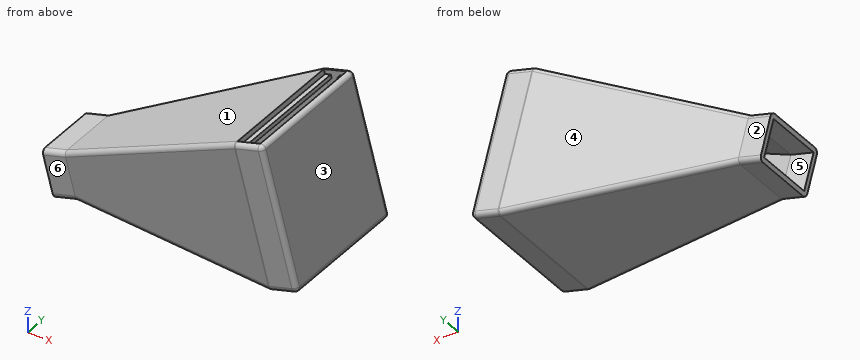
from build123d import *

# Parameters (mm, degrees)
SKETCH037_W             = 110
SKETCH037_H             = 110
PAD002_DEPTH            = 220
POCKET012_DEPTH         = 158
POCKET001_DEPTH         = 158
THICKNESS001_T          = 4
SKETCH014_W             = 110
SKETCH014_H             = 4
POCKET013_DEPTH         = 4
SKETCH016_W             = 3
SKETCH016_H             = 3
PAD022_DEPTH            = 110
SKETCH018_W             = 110
SKETCH018_H             = 16
POCKET014_DEPTH         = 4
SKETCH019_W             = 3
SKETCH019_H             = 5
PAD007_DEPTH            = 110
BODY007_ROLL_ANGLE      = 105
BODY007_PLACEMENT_ANGLE = -90


with BuildPart() as part:
    # Sketch037 → Pad002 (new body)
    with BuildSketch(Plane.XY):
        Rectangle(SKETCH037_W, SKETCH037_H)
    extrude(amount=PAD002_DEPTH)

    # Sketch038 (on Face3 of Pad002) → Pocket012 (cut)
    with BuildSketch(Plane.XZ.offset(55)):
        Polygon((-55, 20), (-25.5, 200), (-25.5, 220), (-55, 220), align=None)
        Polygon((25.5, 220), (55, 220), (55, 20), (25.5, 200), align=None)
    extrude(amount=-POCKET012_DEPTH, mode=Mode.SUBTRACT)

    # Sketch008 (on DatumPlane) → Pocket001 (cut)
    with BuildSketch(Plane.YZ.offset(55)):
        Polygon((-55, 20), (-15.5, 200), (-15.5, 220), (-55, 220), align=None)
        Polygon((15.5, 220), (15.5, 200), (55, 20), (55, 220), align=None)
    extrude(amount=-POCKET001_DEPTH, mode=Mode.SUBTRACT)

    # Thickness001
    thickness001_openings = [part.faces().sort_by_distance(p)[0] for p in [
        (0, 0, 220),
    ]]
    offset(amount=THICKNESS001_T, openings=thickness001_openings)

    # Sketch014 (on Face42 of Thickness001) → Pocket013 (cut)
    with BuildSketch(Plane(origin=(0, 59, 0), x_dir=(-1, 0, 0), z_dir=(0, 1, 0))):
        with Locations((0, 2)):
            Rectangle(SKETCH014_W, SKETCH014_H)
    extrude(amount=-POCKET013_DEPTH, mode=Mode.SUBTRACT)

    # Sketch016 (on Face35 of Pocket013) → Pad022 (join)
    with BuildSketch(Plane(origin=(0, -55, 0), x_dir=(-1, 0, 0), z_dir=(0, 1, 0))):
        with Locations((-53.5, 5.5)):
            Rectangle(SKETCH016_W, SKETCH016_H)
        with Locations((53.5, 5.5)):
            Rectangle(SKETCH016_W, SKETCH016_H)
    extrude(amount=PAD022_DEPTH)

    # Sketch018 (on Face36 of Pad022) → Pocket014 (cut)
    with BuildSketch(Plane(origin=(0, 59, 0), x_dir=(-1, 0, 0), z_dir=(0, 1, 0))):
        with Locations((0, 12)):
            Rectangle(SKETCH018_W, SKETCH018_H)
    extrude(amount=-POCKET014_DEPTH, mode=Mode.SUBTRACT)

    # Sketch019 (on Face49 of Pocket014) → Pad007 (join)
    with BuildSketch(Plane(origin=(55, 0, 0), x_dir=(0, -1, 0), z_dir=(-1, 0, 0))):
        with Locations((-53.5, 17.5)):
            Rectangle(SKETCH019_W, SKETCH019_H)
    extrude(amount=PAD007_DEPTH)


with BuildPart() as part_1:
    # Body007 roll: moved
    add(part.part.rotate(Axis((0, 0, 0), (1, 0, 0)), BODY007_ROLL_ANGLE))


with BuildPart() as part_2:
    # Body007 placement: moved
    add(part_1.part.moved(Location((243.899571, 0, 96.933558))).rotate(Axis((243.899571, 0, 96.933558), (0, 0, 1)), BODY007_PLACEMENT_ANGLE))


solid = part_2.part
Here's how the part is built. I have some questions about the finished solid (model axes, mm). Face numbers are marked on the shaded views. A direction names the side the tool comes from. Coordinates: 2 decimals unless noted, no trailing zeros.
Item 1: On a 3-axis mill with a long thin cutter (end or side, diameter ignored), from which of +Z, -Z, +X, -X, +Y, -Y can I reach the whole of each face in a straight line? I mean the marked faces 1 and 2. Say none if no direction works.
Item 2: If we mould it in two halves opening along Y, with no side actions, what happens to the marked faces 3, 4, 5 and 6? For each: +Y half, -Y half, draft (parallel to the pull), parting line (faces both ways), or undercut.
Item 3: Will these pins go through, and if not, where does the flat tip stop? pin 1 (6 mm diameter, centred on x = 77.5, y = -18, fed in from -Z); pin 2 (1 mm diameter, centred on y = 23, z = 92, fed in from +X); pin 3 (4 mm diameter, centred on y = 36, z = 46, fed in from +X).
Item 4: If I drill on line 1 (Y direction, x = 50, z = 37); line 2 (Z direction, x = 146.5, y = 2); line 3 (X direction, y = -22.5, z = 118.5), over which ranges is the centre line in solid material (lowest first)?
Findings below:
1. face 1: +Z, -X, +Y, -Y
1. face 2: -Z, -X, +Y
2. face 3: draft
2. face 4: +Y half
2. face 5: undercut
2. face 6: -Y half
3. pin 1: stops at z = 27.1
3. pin 2: stops at x = 249.5
3. pin 3: stops at x = 262.13
4. line 1: y = -29.5 to -25.5, 25.5 to 29.5
4. line 2: z = 30.4 to 34.4, 111.82 to 116.33
4. line 3: x = 150.7 to 159.4, 238.12 to 242.26
